from build123d import *

# Parameters (mm, degrees)
SKETCH_1_R      = 1.6
SKETCH_1_R_2    = 31
SKETCH_1_R_3    = 21.1
EXTRUDE_1_DEPTH = 2


with BuildPart() as part:
    # 草图1 → 凸台-拉伸1 (new body)
    # profile 1 of 2: a face of its own
    with BuildSketch(Plane(origin=(0, 0, 0), x_dir=(1, 0, 0), z_dir=(0, 1, 0))):
        with BuildLine():
            Line((-31, 31), (-31, 0))
            ThreePointArc((-31, 0), (0, 31), (31, 0))
            Line((31, 0), (31, 31))
            Line((31, 31), (31, 46))
            Line((31, 46), (-31, 46))
            Line((-31, 46), (-31, 31))
        make_face()
        with Locations(Location((-25, 38.5, 0), (0, 0, 270))):
            Circle(SKETCH_1_R, mode=Mode.SUBTRACT)
        with Locations(Location((0, 38.5, 0), (0, 0, 270))):
            Circle(SKETCH_1_R, mode=Mode.SUBTRACT)
        with Locations(Location((25, 38.5, 0), (0, 0, 270))):
            Circle(SKETCH_1_R, mode=Mode.SUBTRACT)
    # profile 2 of 2: a face of its own
    with BuildSketch(Plane(origin=(0, 0, 0), x_dir=(1, 0, 0), z_dir=(0, 1, 0))):
        Circle(SKETCH_1_R_2)
        with Locations(Location((-18.384776311, 18.384776311, 0), (0, 0, 270))):
            Circle(SKETCH_1_R, mode=Mode.SUBTRACT)
        with Locations(Location((-18.384776311, -18.384776311, 0), (0, 0, 270))):
            Circle(SKETCH_1_R, mode=Mode.SUBTRACT)
        with Locations(Location((18.384776311, -18.384776311, 0), (0, 0, 270))):
            Circle(SKETCH_1_R, mode=Mode.SUBTRACT)
        with Locations(Location((18.384776311, 18.384776311, 0), (0, 0, 270))):
            Circle(SKETCH_1_R, mode=Mode.SUBTRACT)
        with Locations(Location((0, 0, 0), (0, 0, 270))):
            Circle(SKETCH_1_R_3, mode=Mode.SUBTRACT)
    extrude(amount=EXTRUDE_1_DEPTH)


solid = part.part
Input: part model. Units: mm. Frame: model coordinates. Give positions to 0.01 mm unless a question says otherwise; leave off trailing zeros. Loops run counter-clockwise (first coordinate to the right, second up) from the corner with the lowest first, then second, coordinate; pieces in that order, holes last. Notation, with made-up numbers: (77.5, -37.75) - (81.5, -37.75) arc R14 cw to (81.5, -24.75) - close; hole circle Ø11 at (21, 58.25). An arc over 180 degrees is marked (long way). Use CSV: the item, a comma, the result in double quotes. Start each with the question number.
Item 1: Section B-B on z = -38.5. Return loops of the section in (x, y).
Item 2: Section C-C on z = 4.5. Return loops of the section in (x, y), then the cut area to 3 significant figures.
Item 3: Mould query, pull axis Z, two halves, no side actions, for faces 1 (the flat face through (0, 1, -46)), 2 (the flat face through (-31, 1, -23)), 3 (the cylindrical face through (19.97, 0.99, -18.59)). Classes: pulls with the +Z half, pulls with the -Z half, needs draft (parallel to the pull), parting line crosses it, or undercut.
Item 4: Section A-A on x = 0. Return loops of the section in (y, z), then the cut area to 3 significant figures.
Item 5: Line query: line 1 (X direction, y = 1.6, z = -38.5); line 2 (Z direction, x = 17, y = 1.7); line 3 (X direction, y = 0.1, z = 19.5). Output: solid intervals per line, ascending.
Item 6: Section D-D on x = 10. Return loops of the section in (y, z), then the cut area to 3 significant figures.
Ans:
1,outline,"(-31, 0) - (-26.6, 0) - (-26.6, 2) - (-31, 2) - close; (-23.4, 0) - (-1.6, 0) - (-1.6, 2) - (-23.4, 2) - close; (1.6, 0) - (23.4, 0) - (23.4, 2) - (1.6, 2) - close; (26.6, 0) - (31, 0) - (31, 2) - (26.6, 2) - close"
2,outline,"(-30.67, 0) - (-20.61, 0) - (-20.61, 2) - (-30.67, 2) - close; (20.61, 0) - (30.67, 0) - (30.67, 2) - (20.61, 2) - close"
2,area,"40.2 mm2"
3,face 1,"pulls with the -Z half"
3,face 2,"needs draft"
3,face 3,"undercut"
4,outline,"(0, -46) - (2, -46) - (2, -40.1) - (0, -40.1) - close; (0, -36.9) - (2, -36.9) - (2, -21.1) - (0, -21.1) - close; (0, 21.1) - (2, 21.1) - (2, 31) - (0, 31) - close"
4,area,"63.2 mm2"
5,line 1,"x = -31 to -26.6, -23.4 to -1.6, 1.6 to 23.4, 26.6 to 31"
5,line 2,"z = -46 to -19.19, -17.58 to -12.5, 12.5 to 17.58, 19.19 to 25.92"
5,line 3,"x = -24.1 to -19.53, -17.24 to -8.06, 8.06 to 17.24, 19.53 to 24.1"
6,outline,"(0, -46) - (2, -46) - (2, -18.58) - (0, -18.58) - close; (0, 18.58) - (2, 18.58) - (2, 29.34) - (0, 29.34) - close"
6,area,"76.4 mm2"
